Verification items for the finished model (mm, model axes). Give positions to 0.01 mm unless a question says otherwise; leave off trailing zeros. Write each loop counter-clockwise with the first axis right and the second up, starting at its lowest first coordinate (ties: lowest second). Pieces come first, ordered by that corner, then holes. Notation, with made-up numbers: (80.25, 10) -> (124.25, 10) arc R26 cw to (124.25, 24) -> close; hole circle Ø7 at (-19, -1.75). An arc over 180 degrees is marked (long way). Use one line per item in the form item = value. Start each with the question number.
(1) Section check D-D, the plane y = 3.75. State how many separate pieces and enclosed holes the cut face has, plus the area to 3 significant figures.
(2) Depth check by flat-ended pin: pin 1 Ø5.5 at (x, z) = (3.99, -51.51) entering from -Y. Enter the tip coordinate at first touch or a pass-through.
(3) Section check A-A, the plane x = -4.5. Record the cut outline in (y, z).
(4) Section check C-C, the plane z = 0. Record the cut outline in (x, y), plus the area to 3 significant figures.
(5) Section check B-B, the plane z = 60. Record the cut outline in (x, y), plus the area to 3 significant figures.
(6) Scan lines: L1, parallel to Z at x = 15, y = 2.25; L2, parallel to Z at x = -5, y = 5; L3, parallel to X at y = 5, z = -84. Record each from-to range of solid material in increasing order.
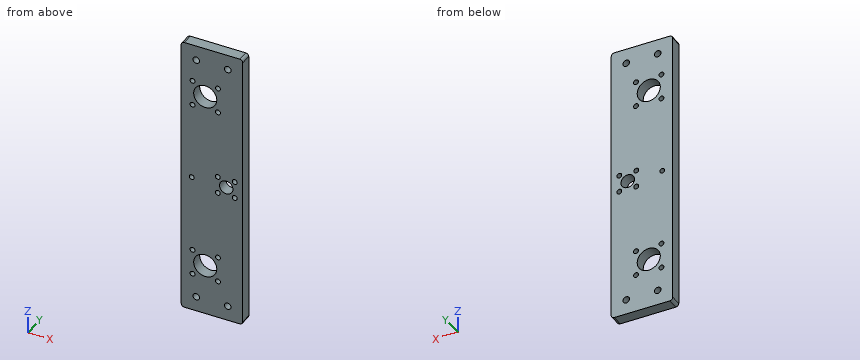
from build123d import *

# Parameters (mm, degrees)
SKETCH1_R           = 2.2
SKETCH1_R_2         = 1.65
SKETCH1_R_3         = 7.7
SKETCH1_R_4         = 4.5
BOSS_EXTRUDE1_DEPTH = 7.5


with BuildPart() as part:
    # Sketch1 → Boss-Extrude1 (new body)
    with BuildSketch(Plane(origin=(0, 7.5, 0), x_dir=(1, 0, 0), z_dir=(0, 1, 0))):
        with BuildLine():
            Line((18.5, 94), (-18.5, 94))
            ThreePointArc((-18.5, 94), (-19.914213562, 93.414213562), (-20.5, 92))
            Line((-20.5, 92), (-20.5, -92))
            ThreePointArc((-20.5, -92), (-19.914213562, -93.414213562), (-18.5, -94))
            Line((-18.5, -94), (18.5, -94))
            ThreePointArc((18.5, -94), (19.914213562, -93.414213562), (20.5, -92))
            Line((20.5, -92), (20.5, 92))
            ThreePointArc((20.5, 92), (19.914213562, 93.414213562), (18.5, 94))
        make_face()
        with Locations((10.5, 84)):
            Circle(SKETCH1_R, mode=Mode.SUBTRACT)
        with Locations((-10.5, 84)):
            Circle(SKETCH1_R, mode=Mode.SUBTRACT)
        with Locations((10.5, -84)):
            Circle(SKETCH1_R, mode=Mode.SUBTRACT)
        with Locations((-10.5, -84)):
            Circle(SKETCH1_R, mode=Mode.SUBTRACT)
        with Locations((3.985281374, 51.514718626)):
            Circle(SKETCH1_R_2, mode=Mode.SUBTRACT)
        with Locations((15.156854249, 5.656854249)):
            Circle(SKETCH1_R_2, mode=Mode.SUBTRACT)
        with Locations((-12.985281374, -68.485281374)):
            Circle(SKETCH1_R_2, mode=Mode.SUBTRACT)
        with Locations((3.985281374, -68.485281374)):
            Circle(SKETCH1_R_2, mode=Mode.SUBTRACT)
        with Locations((-4.5, -60)):
            Circle(SKETCH1_R_3, mode=Mode.SUBTRACT)
        with Locations((9.5, 0)):
            Circle(SKETCH1_R_4, mode=Mode.SUBTRACT)
        with Locations((-12.985281374, -51.514718626)):
            Circle(SKETCH1_R_2, mode=Mode.SUBTRACT)
        with Locations((3.985281374, -51.514718626)):
            Circle(SKETCH1_R_2, mode=Mode.SUBTRACT)
        with Locations((3.985281374, 68.485281374)):
            Circle(SKETCH1_R_2, mode=Mode.SUBTRACT)
        with Locations((-12.985281374, 68.485281374)):
            Circle(SKETCH1_R_2, mode=Mode.SUBTRACT)
        with Locations((-12.985281374, 51.514718626)):
            Circle(SKETCH1_R_2, mode=Mode.SUBTRACT)
        with Locations((3.843145751, 5.656854249)):
            Circle(SKETCH1_R_2, mode=Mode.SUBTRACT)
        with Locations((3.843145751, -5.656854249)):
            Circle(SKETCH1_R_2, mode=Mode.SUBTRACT)
        with Locations((15.156854249, -5.656854249)):
            Circle(SKETCH1_R_2, mode=Mode.SUBTRACT)
        with Locations((-13.5, 0)):
            Circle(SKETCH1_R_2, mode=Mode.SUBTRACT)
        with Locations((-4.5, 60)):
            Circle(SKETCH1_R_3, mode=Mode.SUBTRACT)
    extrude(amount=-BOSS_EXTRUDE1_DEPTH)


solid = part.part
Completed:
q1.separate_pieces = 1
q1.enclosed_holes = 20
q1.area = 7,100 mm²
q2.pin_1 = 0
q3.outline = (0, -94) -> (7.5, -94) -> (7.5, -67.7) -> (0, -67.7) -> close; (0, -52.3) -> (7.5, -52.3) -> (7.5, 52.3) -> (0, 52.3) -> close; (0, 67.7) -> (7.5, 67.7) -> (7.5, 94) -> (0, 94) -> close
q4.outline = (-20.5, 0) -> (-15.15, 0) -> (-15.15, 7.5) -> (-20.5, 7.5) -> close; (-11.85, 0) -> (5, 0) -> (5, 7.5) -> (-11.85, 7.5) -> close; (14, 0) -> (20.5, 0) -> (20.5, 7.5) -> (14, 7.5) -> close
q4.area = 215 mm²
q5.outline = (-20.5, 0) -> (-12.2, 0) -> (-12.2, 7.5) -> (-20.5, 7.5) -> close; (3.2, 0) -> (20.5, 0) -> (20.5, 7.5) -> (3.2, 7.5) -> close
q5.area = 192 mm²
q6.L1 = -94 to -7.3, -4.01 to 4.01, 7.3 to 94
q6.L2 = -94 to -67.68, -52.32 to 52.32, 67.68 to 94
q6.L3 = -20.5 to -12.7, -8.3 to 8.3, 12.7 to 20.5
